Can you work these out from the model? Positions are in its coordinate system, mm. Coordinates: 2 decimals unless noted, no trailing zeros. Write each loop counter-clockwise with the first axis right and the second up, starting at its lowest first coordinate (ties: lowest second). Pieces come first, ordered by that corner, then holes. Notation, with made-up numbers: (86.25, 54.25) -> (145.25, 54.25) arc R12 ccw to (145.25, 66.25) -> close; hole circle Ø5 at (50, 54). An arc over 180 degrees is marked (long way). Use one line per item in the form item = value.
```python
from build123d import *

# Parameters (mm, degrees)
F1_DEPTH = 17.1
F2_R     = 9.8201820523
F3_DEPTH = 25
F5_DEPTH = 34.9
F6_R     = 10
F7_DEPTH = 52.001


with BuildPart() as f1:
    # F0 (on Front) → F1 (new body)
    with BuildSketch(Plane.XZ):
        with BuildLine():
            Line((-18.8324629198, 51.7522737756), (-18.8324629198, -18.2477262244))
            ThreePointArc((-18.8324629198, -18.2477262244), (1.1675370802, -38.2477262244), (21.1675370802, -18.2477262244))
            Line((21.1675370802, -18.2477262244), (21.1675370802, 51.7522737756))
            ThreePointArc((21.1675370802, 51.7522737756), (1.1675370802, 71.7522737756), (-18.8324629198, 51.7522737756))
        make_face()
    extrude(amount=F1_DEPTH)

    # F2 (on face) → F3 (cut)
    with BuildSketch(Plane.XZ.offset(17.1)):
        with Locations((1.1675370802, 51.7522737756)):
            Circle(F2_R)
    extrude(amount=-F3_DEPTH, mode=Mode.SUBTRACT)

    # F4 (on face) → F5 (join)
    with BuildSketch(Plane(origin=(0, 0, 0), x_dir=(-1, 0, 0), z_dir=(0, 1, 0))):
        with BuildLine():
            ThreePointArc((-21.1675370802, -18.2477262244), (-1.1675370802, -38.2477262244), (18.8324629198, -18.2477262244))
            ThreePointArc((18.8324629198, -18.2477262244), (-1.1675370802, 1.7522737756), (-21.1675370802, -18.2477262244))
        make_face()
    extrude(amount=F5_DEPTH)

    # F6 (on face) → F7 (cut, through all)
    with BuildSketch(Plane.XZ.offset(17.1)):
        with Locations((1.1675370802, -18.2477262244)):
            Circle(F6_R)
    extrude(amount=-F7_DEPTH, mode=Mode.SUBTRACT)

    # F8: F1 across face


with BuildPart() as f1_1:
    add(f1.part)
    add(f1.part.mirror(Plane(origin=(1.1675370802, 34.9, -18.2477262244), x_dir=(-1, 0, 0), z_dir=(0, 1, 0))))


solid = f1_1.part
```
Q1. Suppose I cut it at D-D (z = 56). Write out the boundary of the cut face in (x, y), then the cut area to 3 significant figures.
Return value:
outline = (-18.38, -17.1) -> (-7.69, -17.1) -> (-7.69, 0) -> (-18.38, 0) -> close; (-18.38, 69.8) -> (-7.69, 69.8) -> (-7.69, 86.9) -> (-18.38, 86.9) -> close; (10.02, -17.1) -> (20.71, -17.1) -> (20.71, 0) -> (10.02, 0) -> close; (10.02, 69.8) -> (20.71, 69.8) -> (20.71, 86.9) -> (10.02, 86.9) -> close
area = 731 mm2
Q2. Suppose I cut it at A-A (z = 8). Write out the boundary of the cut face in (x, y), then the cut area to 3 significant figures.
Return value:
outline = (-18.83, -17.1) -> (21.17, -17.1) -> (21.17, 0) -> (-18.83, 0) -> close; (-18.83, 69.8) -> (21.17, 69.8) -> (21.17, 86.9) -> (-18.83, 86.9) -> close
area = 1,370 mm2
Q3. If I drill on line 1 (Y direction, x = 11.5, z = 38.5); line 2 (Z direction, x = -7, y = 82.5); line 3 (X direction, y = 77, z = -14), over which ranges is the centre line in solid material (lowest first)? Write a range as from..to.
Return value:
line_1 = -17.1..0, 69.8..86.9
line_2 = -36.5..-24.02, -12.48..46.3, 57.2..70.01
line_3 = -18.83..-7.89, 10.22..21.17
Q4. Thinking about a two-plate mould opening in X: for faces 1 (the flat face through (21.168, 78, 16)), 2 (the cylindrical face through (-0.11, 78.47, 61.49)), 3 (the cylindrical face through (-8.06, 35.63, -35.99)), 4 (the flat face through (1, 69.8, 27)), which applies, released by +X, released by -X, zero draft, split by the parting line, or undercut?
Return value:
face_1 = released by +X
face_2 = undercut
face_3 = split by the parting line
face_4 = zero draft
Q5. Will these pins go through, and if not, where does the flat tip stop? pin 1 (1 mm diameter, centred on y = 45.5, z = -24, fed in from +X); pin 2 (15.5 mm diameter, centred on x = 1.17, z = 51.75, fed in from +Y); pin 3 (10 mm diameter, centred on y = 55.5, z = -9, fed in from -X); pin 4 (3 mm diameter, centred on x = 0.5, y = -6, fed in from +Z).
Return value:
pin_1 = 20.47
pin_2 = through
pin_3 = -18.38
pin_4 = 71.75
Q6. Suppose I cut it at B-B (y = 81). Write out the boundary of the cut face in (x, z).
Return value:
outline = (-18.83, -18.25) arc R20 ccw to (21.17, -18.25) -> (21.17, 51.75) arc R20 ccw to (-18.83, 51.75) -> close; hole circle Ø20 at (1.17, -18.25); hole circle Ø19.64 at (1.17, 51.75)
Q7. Suppose I cut it at C-C (x = -5). Write out the boundary of the cut face in (y, z), then the cut area to 3 significant figures.
Return value:
outline = (-17.1, -37.27) -> (86.9, -37.27) -> (86.9, -26.12) -> (-17.1, -26.12) -> close; (-17.1, -10.38) -> (86.9, -10.38) -> (86.9, 44.11) -> (69.8, 44.11) -> (69.8, 0.78) -> (0, 0.78) -> (0, 44.11) -> (-17.1, 44.11) -> close; (-17.1, 59.39) -> (0, 59.39) -> (0, 70.78) -> (-17.1, 70.78) -> close; (69.8, 59.39) -> (86.9, 59.39) -> (86.9, 70.78) -> (69.8, 70.78) -> close
area = 4,190 mm2
